```python
from build123d import *

# Parameters (mm, degrees)
F1_DEPTH = 6.5
F2_DEPTH = 7.5
F3_DEPTH = 5.25
F0_W     = 0.8
F0_H     = 8
F4_DEPTH = 2.4
F5_SIZE  = 1


with BuildPart() as f1:
    # F0 (on Right) → F1 (new body, symmetric)
    with BuildSketch(Plane.YZ):
        Polygon((8.65, 0), (-8.65, 0), (-8.65, -8.7), (-9.4, -8.7), (-9.4, -14.7), (-7.5, -14.7), (-6.7, -14.7), (-0.4, -14.7), (0.4, -14.7), (6.7, -14.7), (7.5, -14.7), (9.4, -14.7), (9.4, -8.7), (8.65, -8.7), align=None)
    extrude(amount=F1_DEPTH, both=True)

    # F0 (on Right) → F2 (join, symmetric)
    with BuildSketch(Plane.YZ):
        Polygon((-10.5, 2), (-10.5, 0), (-9.4, 0), (-8.65, 0), (8.65, 0), (9.4, 0), (10.5, 0), (10.5, 2), (7.5, 2), (-7.5, 2), align=None)
    extrude(amount=F2_DEPTH, both=True)

    # F0 (on Right) → F3 (join, symmetric)
    with BuildSketch(Plane.YZ):
        with BuildLine():
            ThreePointArc((4.5, 5), (-1.315342, 2.761366), (-7.5, 2))
            Line((-7.5, 2), (7.5, 2))
            Line((7.5, 2), (4.5, 5))
        make_face()
    extrude(amount=F3_DEPTH, both=True)

    # F0 (on Right) → F4 (join, symmetric)
    with BuildSketch(Plane.YZ):
        Polygon((-8.65, 0), (-9.4, 0), (-10.5, -4.35), (-9.4, -8.7), (-8.65, -8.7), (-9.75, -4.35), align=None)
        Polygon((9.4, 0), (8.65, 0), (9.75, -4.35), (8.65, -8.7), (9.4, -8.7), (10.5, -4.35), align=None)
        with Locations((7.1, -18.7)):
            Rectangle(F0_W, F0_H)
        with Locations((0, -18.7)):
            Rectangle(F0_W, F0_H)
        with Locations((-7.1, -18.7)):
            Rectangle(F0_W, F0_H)
    extrude(amount=F4_DEPTH, both=True)

    # F5
    f5_edges = [f1.edges().sort_by_distance(p)[0] for p in [
        (2.4, -7.1, -22.7),
        (2.4, 0, -22.7),
        (-2.4, 7.1, -22.7),
        (2.4, 7.1, -22.7),
        (-2.4, 0, -22.7),
        (-2.4, -7.1, -22.7),
    ]]
    chamfer(f5_edges, length=F5_SIZE)


solid = f1.part
```
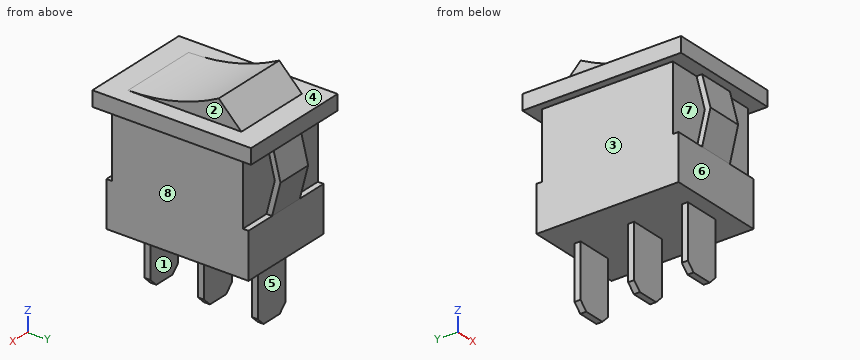
CAD build for the part. Positions are in the model's coordinates, mm. Face numbers are marked on the shaded views. A direction names the side the tool comes from. Round coordinates to 2 decimals unless told otherwise and drop trailing zeros. Order: outer loops, then holes, each group sorted by start corner. A loop starts at its lowest first (then second) coordinate and runs counter-clockwise, first axis right, second up. Notation, with made-up numbers: (-32.5, -35) - (10.5, -35) arc R17 ccw to (10.5, -17) - close; hole circle Ø4 at (17, -16.5). An arc over 180 degrees is marked (long way). Answer in a Markdown table with one row per item. Add a question column.
(1) Band-saw the part on B-B on z = -20.5. List the corners of the cut face in (x, y).
(2) Band-saw the part on D-D on z = -9.75. List the corners of the cut face in (x, y).
(3) Mould opens along Y. For the marked faces 5, 6, 7 and 8 say: +Y half, -Y half, draft (parallel to the pull), parting line (faces both ways), or undercut.
(4) Band-saw the part on C-C on y = 6.25. List the corners of the cut face in (x, z), and give its area (3 significant figures).
(5) Band-saw the part on A-A on x = 3. List the corners of the cut face in (y, z), and give its area (3 significant figures).
(6) Probe L1, parallel to Y at x = 0, z = -18.25; L2, parallel to Y at x = 0, z = -1.75; L3, parallel to Z at x = -2, y = -8.25. List the from-to ranges inside material, lowest first. Write a range as [from, to].
(7) Drop flat-ended pins along their axis: pin 1 Ø8 at (x, y) = (6, -6.5) entering from -Z (3 decimals); pin 2 Ø2 at (y, z) = (-10, -3) entering from +X; pin 3 Ø2 at (x, z) = (3, -18.5) entering from -Y. Give the stop position or say it passes through.
(8) 3-axis set-ups, long thin cutter, end or side, ignore diameter. For the marked faces 1, 2, 3 and 4: which of +Z, -Z, +X, -X, +Y, -Y reach the whole face in a straight line?
Data:
| question | item | result |
|---|---|---|
| 1 | outline | (-2.4, -7.5) - (2.4, -7.5) - (2.4, -6.7) - (-2.4, -6.7) - close; (-2.4, -0.4) - (2.4, -0.4) - (2.4, 0.4) - (-2.4, 0.4) - close; (-2.4, 6.7) - (2.4, 6.7) - (2.4, 7.5) - (-2.4, 7.5) - close |
| 2 | outline | (-6.5, -9.4) - (6.5, -9.4) - (6.5, 9.4) - (-6.5, 9.4) - close |
| 3 | face 5 | +Y half |
| 3 | face 6 | -Y half |
| 3 | face 7 | undercut |
| 3 | face 8 | draft |
| 4 | outline | (-7.5, 0) - (-6.5, 0) - (-6.5, -14.7) - (6.5, -14.7) - (6.5, 0) - (7.5, 0) - (7.5, 2) - (5.25, 2) - (5.25, 3.25) - (-5.25, 3.25) - (-5.25, 2) - (-7.5, 2) - close |
| 4 | area | 234 mm^2 |
| 5 | outline | (-10.5, 0) - (-8.65, 0) - (-8.65, -8.7) - (-9.4, -8.7) - (-9.4, -14.7) - (9.4, -14.7) - (9.4, -8.7) - (8.65, -8.7) - (8.65, 0) - (10.5, 0) - (10.5, 2) - (7.5, 2) - (4.5, 5) arc R25.5 cw to (-7.5, 2) - (-10.5, 2) - close |
| 5 | area | 322 mm^2 |
| 6 | L1 | y = [-7.5, -6.7], [-0.4, 0.4], [6.7, 7.5] |
| 6 | L2 | y = [-9.84, -9.09], [-8.65, 8.65], [9.09, 9.84] |
| 6 | L3 | z = [-14.7, 2] |
| 7 | pin 1 | stops at z = -22.095 |
| 7 | pin 2 | stops at x = 2.4 |
| 7 | pin 3 | stops at y = -7.5 |
| 8 | face 1 | -Z, +X, -X |
| 8 | face 2 | +Z, +X, +Y, -Y |
| 8 | face 3 | -Z, -X, +Y, -Y |
| 8 | face 4 | +Z |
